from build123d import *

# Parameters (mm, degrees)
ESQUISSE1_R                  = 2.5
BASE_EXTRUSION_DEPTH         = 1.5
CONG_1_R                     = 0.8
ESQUISSE2_R                  = 1.25
BOSS_EXTRU_1_DEPTH           = 5
CHANFREIN1_SIZE              = 0.2
ESQUISSE3_W                  = 1
ESQUISSE3_H                  = 1
ENL_V_MAT_EXTRU_1_DEPTH      = 3.5
ENL_V_MAT_EXTRU_1_DEPTH_BACK = 3.5


with BuildPart() as part:
    # Esquisse1 → Base-Extrusion (new body)
    with BuildSketch(Plane.XY):
        Circle(ESQUISSE1_R)
    extrude(amount=BASE_EXTRUSION_DEPTH)

    # Cong_1
    cong_1_edges = [part.edges().sort_by_distance(p)[0] for p in [
        (-2.5, 0, 0),
    ]]
    fillet(cong_1_edges, radius=CONG_1_R)

    # Esquisse2 → Boss.-Extru.1 (add)
    with BuildSketch(Plane.XY.offset(1.5)):
        Circle(ESQUISSE2_R)
    extrude(amount=BOSS_EXTRU_1_DEPTH)

    # Chanfrein1
    chanfrein1_edges = [part.edges().sort_by_distance(p)[0] for p in [
        (-1.25, 0, 6.5),
    ]]
    chamfer(chanfrein1_edges, length=CHANFREIN1_SIZE)

    # Esquisse3 → Enl_v. mat.-Extru.1 (cut, two sides)
    with BuildSketch(Plane(origin=(0, 0, 0), x_dir=(1, 0, 0), z_dir=(0, 1, 0))) as enl_v_mat_extru_1_sk:
        with Locations((0, -0.5)):
            Rectangle(ESQUISSE3_W, ESQUISSE3_H)
    extrude(amount=ENL_V_MAT_EXTRU_1_DEPTH, mode=Mode.SUBTRACT)
    extrude(enl_v_mat_extru_1_sk.sketch, amount=-ENL_V_MAT_EXTRU_1_DEPTH_BACK, mode=Mode.SUBTRACT)


solid = part.part
Can you work these out from the model? Positions are in its coordinate system, mm. A direction names the side the tool comes from. Give positions to 0.01 mm unless a question says otherwise; leave off trailing zeros. Loops run counter-clockwise (first coordinate to the right, second up) from the corner with the lowest first, then second, coordinate; pieces in that order, holes last. Notation, with made-up numbers: M 1.5,86.25 L 22.5,86.25 A33 cw 22.5,124.25 Z; hole C 49,-0.75 d2. An arc over 180 degrees is marked long. One line per item, written item: value. Start each with the question number.
1) I'm going to push flat-ended pins straight in: pin 1 (1.5 mm diameter, centred on x = -1, z = 4, fed in from -Y); pin 2 (2 mm diameter, centred on x = -2, y = 2, fed in from -Z); pin 3 (1.1 mm diameter, centred on y = 1, z = 0.5, fed in from +X). Where does each tip first touch, or does it pass through?
2) If we section it at A-A, the plane y = 0: Write out the boundary of the cut face in (x, z), and give its area (3 significant figures).
3) If I drill on line 1 (Y direction, x = -0.05, z = 3.5); line 2 (Z direction, x = -0.85, y = -1.4); line 3 (Y direction, x = 0.9, z = 1.25), over which ranges is the centre line in solid material (lowest first)? Write a range as [from, to].
4) If we section it at C-C, the plane z = 3: Write out the boundary of the cut face in (x, y), and give its area (3 significant figures).
5) Thinking about a two-plate mould opening in X: for faces 4 (the face through (-0.5, 0, 0.5)), 5 (the face through (0, 0, 6.5)), 6 (the face through (-0.27, -1.22, 3.87)), which applies, +X half, -X half, draft (parallel to the pull), parting line (faces both ways), or undercut?
6) If we section it at B-B, the plane x = 0: Write out the boundary of the cut face in (y, z), and give its area (3 significant figures).
7) On a 3-axis mill with a long thin cutter (end or side, diameter ignored), from which of +Z, -Z, +X, -X, +Y, -Y can I reach the whole of each face in a straight line? I mean faces 1 (the face through (-0.54, -2.44, 1.15)), 2 (the face through (0.5, 0, 0.5)), 3 (the face through (-1, -1, 1.5)). Say none if no direction works.
Completed:
1. pin 1: stops at y = -1.22
1. pin 2: stops at z = 0.01
1. pin 3: stops at x = 2.45
2. outline: M -2.5,0.8 A0.8 ccw -1.7,0 L -0.5,0 L -0.5,1 L 0.5,1 L 0.5,0 L 1.7,0 A0.8 ccw 2.5,0.8 L 2.5,1.5 L 1.25,1.5 L 1.25,6.3 L 1.05,6.5 L -1.05,6.5 L -1.25,6.3 L -1.25,1.5 L -2.5,1.5 Z
2. area: 18.7 mm^2
3. line 1: y = [-1.25, 1.25]
3. line 2: z = [0, 1.5]
3. line 3: y = [-2.33, 2.33]
4. outline: C 0,0 d2.5
4. area: 4.91 mm^2
5. face 4: undercut
5. face 5: draft
5. face 6: parting line
6. outline: M -2.5,1 L 2.5,1 L 2.5,1.5 L 1.25,1.5 L 1.25,6.3 L 1.05,6.5 L -1.05,6.5 L -1.25,6.3 L -1.25,1.5 L -2.5,1.5 Z
6. area: 15.0 mm^2
7. face 1: +Z, -Z
7. face 2: -Z, +Y, -Y
7. face 3: +Z
